Geometry check sheet. Reference: the model listing, model coordinates, mm. Face numbers are marked on the shaded views. Round coordinates to 2 decimals unless told otherwise and drop trailing zeros. Loops run counter-clockwise (first coordinate to the right, second up) from the corner with the lowest first, then second, coordinate; pieces in that order, holes last.
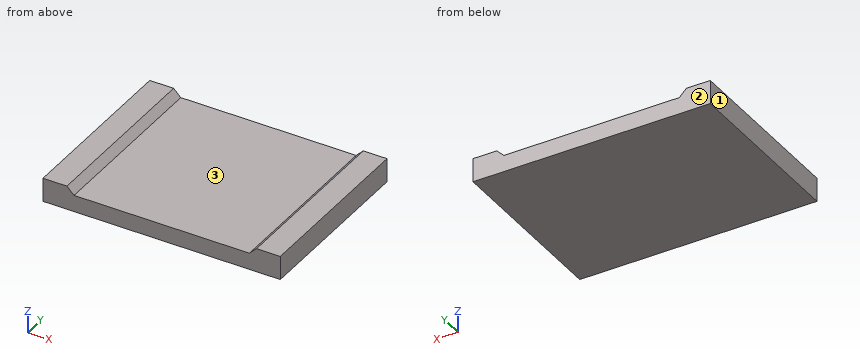
Autodesk Inventor part; units mm, degrees
ref_plane "YZ Plane" through (0, 0, 0) normal (1, 0, 0) x (0, 1, 0)
ref_plane "XZ Plane" through (0, 0, 0) normal (0, 1, 0) x (-1, 0, 0)
ref_plane "XY Plane" through (0, 0, 0) normal (0, 0, 1) x (1, 0, 0)
sketch "Sketch1" plane through (0, 0, 0) normal (0, 1, 0) x (-1, 0, 0)
  line L0 (100, 0) -> (100, -10)
  line L1 (100, -10) -> (0, -10)
  line L2 (0, -10) -> (0, 0)
  line L3 (0, 0) -> (10, 0)
  line L4 (13, -3) -> (10, 0)
  line L5 (86.9207, -3) -> (89.9207, 0)
  line L6 (13, -3) -> (86.9207, -3)
  line L7 (0, 0) -> (10, 0)
  line L8 (89.9207, 0) -> (100, 0)
  point P0 (13, 0)
  point P1 (13, 0)
  point P2 (89.9207, 0)
  point P3 (89.9207, 0)
  point P4 (86.9207, 0)
extrude "Extrusion1" add sketch "Sketch1" along normal blind 75
sketch "Sketch2" plane through (0, 0, -10) normal (0, 0, -1) x (-1, 0, 0)
  line L0 (0, 0) -> (100, 0)
  line L1 (100, 0) -> (100, 75)
  line L2 (0, 75) -> (100, 75)
  line L3 (0, 0) -> (0, 75)
properties part number "base" material "Gravel"
1) Mould release check, pull along X, two halves, no side actions. Record for the marked faces 1, 2 and 3: +X half, -X half, draft (parallel to the pull), parting line (faces both ways), or undercut.
Report:
face 1: -X half
face 2: draft
face 3: undercut
2) Sectioned sample at A-A, the plane y = 6. Record the cut outline in (x, z).
Report:
outline: (-100, -10) - (0, -10) - (0, 0) - (-10, 0) - (-13, -3) - (-86.92, -3) - (-89.92, 0) - (-100, 0) - close
3) Scan lines: line 1 along Z through (x, y) = (-84, 58); line 2 along X through (y, z) = (49, -2.5); line 3 along X through (y, z) = (36.5, -1.75). Record each from-to range of solid material in increasing order.
Report:
line 1: z = -10 to -3
line 2: x = -100 to -87.42, -12.5 to 0
line 3: x = -100 to -88.17, -11.75 to 0
4) Sectioned sample at B-B, the plane x = -38.5. Record the cut outline in (y, z), then the cut area to 3 significant figures.
Report:
outline: (0, -10) - (75, -10) - (75, -3) - (0, -3) - close
area: 525 mm2
